from build123d import *

# Parameters (mm, degrees)
BOSS_EXTRUDE1_DEPTH         = 3.175
BOSS_EXTRUDE1_DRAFT         = -28
CUT_EXTRUDE3_DEPTH          = 4.175
BOSS_EXTRUDE2_DEPTH         = 3.175
F_1_4_0_25_DIAMETER_HOLE1_D = 6.35
SKETCH9_R                   = 9.906
SKETCH9_R_2                 = 7.62
CUT_EXTRUDE4_DEPTH          = 4.175
F_1_4_0_25_DIAMETER_HOLE2_D = 6.35


with BuildPart() as part:
    # Sketch1 → Boss-Extrude1 (with draft: the straight prism first)
    with BuildSketch(Plane.XY):
        with BuildLine():
            Line((-101.780957474, 0), (-12.02943471, -167.25772623))
            ThreePointArc((-12.02943471, -167.25772623), (0, -164.234100952), (12.02943471, -167.25772623))
            Line((12.02943471, -167.25772623), (101.780957474, 0))
            Line((101.780957474, 0), (-101.780957474, 0))
        make_face()
    extrude(amount=BOSS_EXTRUDE1_DEPTH)
    # Boss-Extrude1: the draft: its side faces are tilted about the plane it starts from
    boss_extrude1_sides = [part.faces().sort_by_distance(p)[0] for p in [
        (56.905196092, -83.628863115, 1.5875),
        (0, 0, 1.5875),
        (-56.905196092, -83.628863115, 1.5875),
        (0, -164.234100952, 1.5875),
    ]]
    draft(boss_extrude1_sides, Plane.XY, BOSS_EXTRUDE1_DRAFT)

    # Sketch6 → Cut-Extrude3 (cut, through all)
    with BuildSketch(Plane.XY.offset(3.175)):
        Polygon((-103.696831485, 0), (-101.780957474, 0), (101.780957474, 0), (103.696831485, 0), (104.602717866, 1.688177446), (-104.602717866, 1.688177446), align=None)
        with BuildLine():
            Line((-11.231210531, -168.745268245), (-101.780957474, 0))
            Line((-101.780957474, 0), (-103.696831485, 0))
            Line((-103.696831485, 0), (-12.690350956, -169.596420612))
            ThreePointArc((-12.690350956, -169.596420612), (-11.968349556, -169.157869126), (-11.231210531, -168.745268245))
        make_face()
        with BuildLine():
            Line((103.696831485, 0), (101.780957474, 0))
            Line((101.780957474, 0), (11.231210531, -168.745268245))
            ThreePointArc((11.231210531, -168.745268245), (11.968349556, -169.157869126), (12.690350956, -169.596420612))
            Line((12.690350956, -169.596420612), (103.696831485, 0))
        make_face()
    extrude(amount=-CUT_EXTRUDE3_DEPTH, mode=Mode.SUBTRACT)

    # Sketch8 → Boss-Extrude2 (add)
    with BuildSketch(Plane.XY.offset(3.175)):
        Polygon((-101.780957474, 0), (-152.580957474, 0), (-152.580957474, -63.5), (-67.706467619, -63.5), align=None)
        Polygon((152.580957474, -63.5), (67.706467619, -63.5), (101.780957474, 0), (152.580957474, 0), align=None)
    extrude(amount=-BOSS_EXTRUDE2_DEPTH)

    # 1/4 (0.25) Diameter Hole1 (through all)
    with Locations(Plane.XY.offset(3.175)):
        with Locations((-33.3375, -19.05), (-23.8125, -19.05), (-14.2875, -19.05), (-4.7625, -19.05)):
            f_1_4_0_25_diameter_hole1 = Hole(F_1_4_0_25_DIAMETER_HOLE1_D / 2)

    # Mirror1: 1/4 (0.25) Diameter Hole1 across plane
    add(f_1_4_0_25_diameter_hole1.mirror(Plane(origin=(0, 0, 0), x_dir=(0, 0, 1), z_dir=(1, 0, 0))), mode=Mode.SUBTRACT)

    # Sketch9 → Cut-Extrude4 (cut, through all)
    with BuildSketch(Plane.XY.offset(3.175)):
        with Locations((125.639722953, -42.830834866)):
            Circle(SKETCH9_R)
        with Locations((140.652136328, -14.854238493)):
            Circle(SKETCH9_R_2)
        with Locations((113.178020253, -19.05)):
            Circle(SKETCH9_R_2)
        with Locations((98.165606878, -47.026596374)):
            Circle(SKETCH9_R_2)
    extrude(amount=-CUT_EXTRUDE4_DEPTH, mode=Mode.SUBTRACT)

    # 1/4 (0.25) Diameter Hole2 (through all)
    with Locations(Plane.XY.offset(3.175)):
        with Locations((-31.75, -69.85), (-15.875, -69.85), (0, -69.85), (15.875, -69.85), (31.75, -69.85)):
            Hole(F_1_4_0_25_DIAMETER_HOLE2_D / 2)


solid = part.part
Source: CAD feature listing. Evaluate the final solid. Frame: model axes, mm. Round coordinates to 2 decimals unless told otherwise and drop trailing zeros. Loops run counter-clockwise (first coordinate to the right, second up) from the corner with the lowest first, then second, coordinate; pieces in that order, holes last. Notation, with made-up numbers: (-17.75, 73.25) - (-2.75, 73.25) arc R13 cw to (-2.75, 79.25) - close; hole circle Ø6 at (58, -38). An arc over 180 degrees is marked (long way). Write item = value, one per line. Start each with the question number.
(1) Section query A-A, the plane z = 2.3. State how many separate pieces and enclosed holes the cut face has, plus the area to 3 significant figures.
(2) Ray query, line 1 along Y through (x, z) = (15.5, 2.4); line 2 along Y through (x, z) = (-100, 0.75); line 3 along Y through (x, z) = (17, 1). Return the intervals inside material, ascending. Write a range as from..to.
(3) Section query B-B, the plane x = 98. Output: boundary loops of the cut face in (y, z) (3 decimals).
(4) Section query C-C, the plane y = -69.85. Output: boundary loops of the cut face in (x, z) (3 decimals).
(5) Pin query (flat end, axial travel): pin 1 (1 mm diameter, centred on x = 124, z = 1.5, fed in from -Y). Return the tip coordinate at first contact, or that it passes through.
(6) Section query D-D, the plane x = -77. Output: boundary loops of the cut face in (y, z) (3 decimals), plus the area to 3 significant figures.
(7) Pull-direction query (X, two-part tool) for faces 1 (the face through (-39, -117, 2)), 2 (the face through (39.86, -115.39, 1.61)), 3 (the face through (-2, -45, 0)), 4 (the face through (-7.79, -18.1, 1.57)); classes: +X half, -X half, draft (parallel to the pull), parting line (faces both ways), or undercut.
Conclusion:
q1.separate_pieces = 1
q1.enclosed_holes = 17
q1.area = 26,400 mm2
q2.line_1 = -160.79..-73, -66.7..-21.98, -16.12..0
q2.line_2 = -63.5..0
q2.line_3 = -157.99..-72.82, -66.88..-20.7, -17.4..0
q3.outline = (-63.5, 0) - (-54.645, 0) - (-54.645, 3.175) - (-63.5, 3.175) - close; (-39.408, 0) - (0, 0) - (0, 3.175) - (-39.408, 3.175) - close
q4.outline = (-64.299, 0) - (-34.925, 0) - (-34.925, 3.175) - (-64.299, 3.175) - close; (-28.575, 0) - (-19.05, 0) - (-19.05, 3.175) - (-28.575, 3.175) - close; (-12.7, 0) - (-3.175, 0) - (-3.175, 3.175) - (-12.7, 3.175) - close; (3.175, 0) - (12.7, 0) - (12.7, 3.175) - (3.175, 3.175) - close; (19.05, 0) - (28.575, 0) - (28.575, 3.175) - (19.05, 3.175) - close; (34.925, 0) - (64.299, 0) - (64.299, 3.175) - (34.925, 3.175) - close
q5.pin_1 = -63.5
q6.outline = (-63.5, 0) - (0, 0) - (0, 3.175) - (-63.5, 3.175) - close
q6.area = 202 mm2
q7.face_1 = -X half
q7.face_2 = +X half
q7.face_3 = draft
q7.face_4 = undercut
